Geometry check sheet. Reference: the model listing, model coordinates, mm. A direction names the side the tool comes from. Coordinates: 2 decimals unless noted, no trailing zeros. Write each loop counter-clockwise with the first axis right and the second up, starting at its lowest first coordinate (ties: lowest second). Pieces come first, ordered by that corner, then holes. Notation, with made-up numbers: M 28,43.25 L 60,43.25 A22 cw 60,54.25 Z; hole C 40,-37 d1. An arc over 180 degrees is marked long. Write item = value, one per line. Start each with the question number.
```python
from build123d import *

# Parameters (mm, degrees)
F3_R     = 1
F4_DEPTH = 1
F5_DEPTH = 2.86


with BuildPart() as f2:
    # F0 (on Front) → F2 (revolve)
    with BuildSketch(Plane.XZ):
        Polygon((-24.2083683173, 5.8015905717), (-25.5083683173, 5.8015905717), (-25.5083683173, 0.8515905717), (-24.1083683173, 0.8515905717), (-24.1083683173, 0.0015905717), (-19.6583683173, 0.0015905717), (-19.6583683173, 0.7215905717), (-15.0083683173, 0.7215905717), (-15.0083683173, 3.5815905717), (-24.2083683173, 3.5815905717), align=None)
    revolve(axis=Axis((0, 0, 5), (0, 0, -1)))

    # F3 (on face) → F4 (cut)
    with BuildSketch(Plane.XY.offset(3.5815905717)):
        with BuildLine():
            Line((14.8745124138, -2), (17.5083683173, -2))
            ThreePointArc((17.5083683173, -2), (19.5083683173, 0), (17.5083683173, 2))
            Line((17.5083683173, 2), (14.8745124138, 2))
            ThreePointArc((14.8745124138, 2), (14.9748669509, 1.0022371729), (15.0083683173, 0))
            ThreePointArc((15.0083683173, 0), (14.9748669509, -1.0022371729), (14.8745124138, -2))
        make_face()
        with Locations((17.5083683173, 0)):
            Circle(F3_R, mode=Mode.SUBTRACT)
    extrude(amount=-F4_DEPTH, mode=Mode.SUBTRACT)

    # F3 (on face) → F5 (cut)
    with BuildSketch(Plane.XY.offset(3.5815905717)):
        with Locations((17.5083683173, 0)):
            Circle(F3_R)
    extrude(amount=-F5_DEPTH, mode=Mode.SUBTRACT)


solid = f2.part
```
Q1. Gauge pin test, flat ends, axial feed: pin 1 (2.5 mm diameter, centred on x = 17.51, y = 0, fed in from -Z); pin 2 (24 mm diameter, centred on x = -7.5, y = 8.5, fed in from +Z); pin 3 (1.5 mm diameter, centred on y = 10, z = 3, fed in from -X); pin 4 (8 mm diameter, centred on x = 19, y = -14, fed in from +Z). Record the tip position at first contact, or that the pin passes through.
Q2. Cross-section at C-C on z = 1.45. Enter the section's corners in (x, y), and give its area (3 significant figures).
Q3. Set-up check for faces 1 (the face through (18.432, -0.383, 1.665)), 2 (the face through (19.508, -0.044, 3.089)), 3 (the face through (-6, -14, 0.722)): record each of +Z, -Z, +X, -X, +Y, -Y from which the full face is reachable in a straight line by a thin tool's end or side.
Q4. Cross-section at D-D on y = -22. Enter the section's corners in (x, z), and give its area (3 significant figures).
Q5. Cross-section at B-B on y = 0. Enter the section's corners in (x, z), and give its area (3 significant figures).
Q6. Cross-section at A-A on x = 0. Enter the section's corners in (y, z).
Q7. Scan lines: L1, parallel to Y at x = 0, z = 4.6; L2, parallel to Y at x = 0, z = 0.55; L3, parallel to Z at x = 18.5, y = -4.5. Record each from-to range of solid material in increasing order.
Q8. Draft check along Y on faces 4 (the face through (-11.1, -21.4, 0.4)), 5 (the face through (23, -9, 5.802)), 6 (the face through (-18.751, 5.905, 0.367)). Enter one of: pulls with the +Y half, pulls with the -Y half, needs draft (parallel to the pull), parting line crosses it, or undercut.
Values found:
q1.pin_1 = 0.72
q1.pin_2 = 3.58
q1.pin_3 = -23.77
q1.pin_4 = 5.8
q2.outline = C 0,0 d51.02; hole C 0,0 d30.02; hole C 17.51,0 d2
q2.area = 1,330 mm²
q3.face_1 = +Z, -Z
q3.face_2 = +Z
q3.face_3 = -Z
q4.outline = M -12.91,0.85 L -9.86,0.85 L -9.86,0 L 9.86,0 L 9.86,0.85 L 12.91,0.85 L 12.91,5.8 L 10.1,5.8 L 10.1,3.58 L -10.1,3.58 L -10.1,5.8 L -12.91,5.8 Z
q4.area = 99.7 mm²
q5.outline = M -25.51,0.85 L -24.11,0.85 L -24.11,0 L -19.66,0 L -19.66,0.72 L -15.01,0.72 L -15.01,3.58 L -24.21,3.58 L -24.21,5.8 L -25.51,5.8 Z; M 15.01,0.72 L 16.51,0.72 L 16.51,2.58 L 15.01,2.58 Z; M 18.51,0.72 L 19.66,0.72 L 19.66,0 L 24.11,0 L 24.11,0.85 L 25.51,0.85 L 25.51,5.8 L 24.21,5.8 L 24.21,3.58 L 19.51,3.58 L 19.51,2.58 L 18.51,2.58 Z
q5.area = 63.7 mm²
q6.outline = M -25.51,0.85 L -24.11,0.85 L -24.11,0 L -19.66,0 L -19.66,0.72 L -15.01,0.72 L -15.01,3.58 L -24.21,3.58 L -24.21,5.8 L -25.51,5.8 Z; M 15.01,0.72 L 19.66,0.72 L 19.66,0 L 24.11,0 L 24.11,0.85 L 25.51,0.85 L 25.51,5.8 L 24.21,5.8 L 24.21,3.58 L 15.01,3.58 Z
q7.L1 = -25.51 to -24.21, 24.21 to 25.51
q7.L2 = -24.11 to -19.66, 19.66 to 24.11
q7.L3 = 0.72 to 3.58
q8.face_4 = parting line crosses it
q8.face_5 = needs draft
q8.face_6 = undercut
